Can you work these out from the model? Positions are in its coordinate system, mm. A direction names the side the tool comes from. Round coordinates to 2 decimals unless told otherwise and drop trailing zeros. Loops run counter-clockwise (first coordinate to the right, second up) from the corner with the lowest first, then second, coordinate; pieces in that order, holes last. Notation, with made-up numbers: (87, 25) - (129, 25) arc R16 cw to (129, 29) - close; hole circle Ø10 at (-40, 65.25). An arc over 180 degrees is marked (long way). Answer as CSV lines item,"result".
```python
from build123d import *

# Parameters (mm, degrees)
F0_W     = 300
F0_H     = 200
F1_DEPTH = 16
F3_DEPTH = 16


with BuildPart() as f1:
    # F0 (on Right) → F1 (new body)
    with BuildSketch(Plane.YZ):
        with Locations((150, 100)):
            Rectangle(F0_W, F0_H)
    extrude(amount=F1_DEPTH)

    # F2 (on face) → F3 (join)
    with BuildSketch(Plane(origin=(0, 0, 0), x_dir=(0, -1, 0), z_dir=(-1, 0, 0))):
        Polygon((-210, 207), (-210, 200), (-90, 200), (-90, 214), (-150, 214), (-150, 207), align=None)
    extrude(amount=-F3_DEPTH)


solid = f1.part
```
Q1. Imagine slicing it at C-C (y = 280). Write out the boundary of the cut face in (x, z).
Checks:
outline,"(0, 0) - (16, 0) - (16, 200) - (0, 200) - close"
Q2. On a 3-axis mill with a long thin cutter (end or side, diameter ignored), from which of +Z, -Z, +X, -X, +Y, -Y can I reach the whole of each face in a straight line? I mean faces 1 (the flat face through (8, 120, 214)), 2 (the flat face through (8, 90, 207)), 3 (the flat face through (8, 254, 200)). Say none if no direction works.
Checks:
face 1,"+Z, +X, -X, +Y, -Y"
face 2,"+Z, +X, -X, -Y"
face 3,"+Z, +X, -X, +Y"
Q3. If I drill on line 1 along Z through (x, y) = (2.25, 164); line 2 along Z through (x, y) = (6.5, 35); line 3 along Y through (x, z) = (7.5, 202.5), over which ranges is the centre line in solid material (lowest first)? Write a range as [from, to].
Checks:
line 1,"[0, 207]"
line 2,"[0, 200]"
line 3,"[90, 210]"
Q4. Imagine slicing it at B-B (y = 206). Write out the boundary of the cut face in (x, z), then the cut area to 3 significant figures.
Checks:
outline,"(0, 0) - (16, 0) - (16, 207) - (0, 207) - close"
area,"3,310 mm²"
Q5. Imagine slicing it at A-A (x = 8.5). Write out the boundary of the cut face in (y, z).
Checks:
outline,"(0, 0) - (300, 0) - (300, 200) - (210, 200) - (210, 207) - (150, 207) - (150, 214) - (90, 214) - (90, 200) - (0, 200) - close"
Q6. I'm going to push flat-ended pins straight in: pin 1 Ø2 at (x, z) = (5.5, 203) entering from +Y; pin 2 Ø5 at (x, y) = (11, 187) entering from +Z; pin 3 Ø12 at (y, z) = (142.5, 160.5) entering from -X; pin 4 Ø2 at (x, z) = (9.5, 210) entering from +Y. Where does each tip first touch, or does it pass through?
Checks:
pin 1,"y = 210"
pin 2,"z = 207"
pin 3,"x = 0"
pin 4,"y = 150"
